The model under review builds one solid part; all positions refer to its coordinate system, in mm. A direction names the side the tool comes from. Coordinates: 2 decimals unless noted, no trailing zeros. Write each loop counter-clockwise with the first axis right and the second up, starting at its lowest first coordinate (ties: lowest second). Pieces come first, ordered by that corner, then holes.
1) Mouldability with a two-part tool opening along Y and no side actions: class faces 3 (the flat face through (0, 10, 246)), 4 (the flat face through (0, 8, 246)), 5 (the flat face through (0, -10, 246)), 6 (the flat face through (-9, 0, 0)) as released by +Y, released by -Y, zero draft, split by the parting line, or undercut.
2) For line 1 (Y direction, x = -9.2, z = 250); line 2 (X direction, y = 7.25, z = 399), list the stretches that pass through material, from the lowest coordinate up.
3) Machinability: for faces 1 (the flat face through (-10, 0, 246)), 2 (the flat face through (0, -8, 246)), which of the approach directions +Z, -Z, +X, -X, +Y, -Y give a long, thin tool a straight path to every point of the face, cutting with its end or side? Answer none if there is none.
4) Add section A-A, the plane x = 1.5. State the section outline as (y, z) points.
5) Add section B-B, the plane z = 375.5. State the section outline as (x, y) points.
from build123d import *

# Parameters (mm, degrees)
SKETCH1_W           = 20
SKETCH1_H           = 20
SKETCH1_W_2         = 16
SKETCH1_H_2         = 16
BOSS_EXTRUDE1_DEPTH = 500
SKETCH3_R           = 3
CUT_EXTRUDE1_DEPTH  = 501.49975025
LPATTERN1_COUNT     = 9
LPATTERN1_PITCH     = 50


with BuildPart() as part:
    # Sketch1 → Boss-Extrude1 (new body)
    with BuildSketch(Plane.XY):
        Rectangle(SKETCH1_W, SKETCH1_H)
        Rectangle(SKETCH1_W_2, SKETCH1_H_2, mode=Mode.SUBTRACT)
    extrude(amount=BOSS_EXTRUDE1_DEPTH)

    # Sketch3 → Cut-Extrude1 (cut, through all)
    with BuildSketch(Plane.ZY.offset(10)):
        with Locations(Location((50, 0, 0), (0, 0, 270))):
            Circle(SKETCH3_R)
    cut_extrude1 = extrude(amount=-CUT_EXTRUDE1_DEPTH, mode=Mode.SUBTRACT)

    # LPattern1: Cut-Extrude1 ×9
    with Locations(*[(0, 0, i * LPATTERN1_PITCH) for i in range(1, LPATTERN1_COUNT)]):
        add(cut_extrude1, mode=Mode.SUBTRACT)


solid = part.part
Geometry results:
1. face 3: released by +Y
1. face 4: undercut
1. face 5: released by -Y
1. face 6: zero draft
2. line 1: y = -10 to -3, 3 to 10
2. line 2: x = -10 to -8, 8 to 10
3. face 1: +Z, -Z, -X, +Y, -Y
3. face 2: +Z, -Z
4. outline: (-10, 0) - (-8, 0) - (-8, 500) - (-10, 500) - close; (8, 0) - (10, 0) - (10, 500) - (8, 500) - close
5. outline: (-10, -10) - (10, -10) - (10, 10) - (-10, 10) - close; hole (-8, -8) - (8, -8) - (8, 8) - (-8, 8) - close
